from build123d import *

# Parameters (mm, degrees)
BOSS_EXTRUDE1_DEPTH = 10


with BuildPart() as part:
    # Sketch1 → Boss-Extrude1 (new body)
    with BuildSketch(Plane.XY):
        with BuildLine():
            Line((-9.709376273, 1.641432906), (-9.709376273, -21.269563621))
            Line((-9.709376273, -21.269563621), (-4.709376273, -21.269563621))
            Line((-4.709376273, -21.269563621), (-4.709376273, -13.269563621))
            Line((-4.709376273, -13.269563621), (14.600623727, -13.269563621))
            Line((14.600623727, -13.269563621), (14.600623727, -11.159563621))
            ThreePointArc((14.600623727, -11.159563621), (2.126806638, -7.715324743), (-6.812431614, 1.641432906))
            Line((-6.812431614, 1.641432906), (-9.709376273, 1.641432906))
        make_face()
        with BuildLine():
            Line((14.600623727, -11.159563621), (14.600623727, -13.269563621))
            Line((14.600623727, -13.269563621), (33.910623727, -13.269563621))
            Line((33.910623727, -13.269563621), (33.910623727, -21.269563621))
            Line((33.910623727, -21.269563621), (38.910623727, -21.269563621))
            Line((38.910623727, -21.269563621), (38.910623727, 1.641432906))
            Line((38.910623727, 1.641432906), (36.013679069, 1.641432906))
            ThreePointArc((36.013679069, 1.641432906), (27.074440817, -7.715324743), (14.600623727, -11.159563621))
        make_face()
    extrude(amount=BOSS_EXTRUDE1_DEPTH)

    # Sketch4 → CSK for M2 Countersunk Flat Head Screw1 (revolve, cut)
    with BuildSketch(Plane(origin=(-4.709376273, -17.301406974, 5), x_dir=(0, 0, -1), z_dir=(0, 1, 0))):
        Polygon((0, 0), (0, 17.221032743), (1.2, 16.5), (1.2, 1), (2.2, 0), align=None)
    csk_for_m2_countersunk_flat_head_screw1 = revolve(axis=Axis((1.640623727, -17.301406974, 5), (-1, 0, 0)), mode=Mode.SUBTRACT)

    # Mirror2: CSK for M2 Countersunk Flat Head Screw1 across plane
    add(csk_for_m2_countersunk_flat_head_screw1.mirror(Plane(origin=(14.600623727, 0, 0), x_dir=(0, 0, 1), z_dir=(1, 0, 0))), mode=Mode.SUBTRACT)


solid = part.part
The model under review builds one solid part; all positions refer to its coordinate system, in mm. A direction names the side the tool comes from. Round coordinates to 2 decimals unless told otherwise and drop trailing zeros. Order: outer loops, then holes, each group sorted by start corner. A loop starts at its lowest first (then second) coordinate and runs counter-clockwise, first axis right, second up. Notation, with made-up numbers: (12, 17.25) - (43, 17.25) arc R17 ccw to (43, 23.25) - close; hole circle Ø8 at (55, 11.25). An arc over 180 degrees is marked (long way). Use one line per item in the form item = value.
Q1. Clearance check with flat-ended pins moving along their axes: P1, Ø1.4, axis at y = -17.3, z = 5, coming from the -X side; P2, Ø1.5, axis at x = 6, z = 8, coming from the -Y side. State where each tip first meets the part, or that it passes through.
Response values:
P1 = through
P2 = -13.27
Q2. Mouldability with a two-part tool opening along X and no side actions: class faces 1 (the flat face through (-9.709, -10, 5)), 2 (the flat face through (38.911, -10, 5)), 3 (the flat face through (14, -12, 0)), 4 (the flat face through (33.911, -15, 4)) as pulls with the +X half, pulls with the -X half, needs draft (parallel to the pull), parting line crosses it, or undercut.
Response values:
face_1 = pulls with the -X half
face_2 = pulls with the +X half
face_3 = needs draft
face_4 = undercut
Q3. Add section C-C on z = 7.75. Give the boundary of the cut face in (x, y), then the cut area to 3 significant figures.
Response values:
outline = (-9.71, -21.27) - (-4.71, -21.27) - (-4.71, -13.27) - (33.91, -13.27) - (33.91, -21.27) - (38.91, -21.27) - (38.91, 1.64) - (36.01, 1.64) arc R24.31 cw to (-6.81, 1.64) - (-9.71, 1.64) - close
area = 415 mm^2
Q4. Tool access review of faces 5 (the flat face through (-4.709, -18.2, 2.7)), 6 (the flat face through (36, -21.27, 5)): name each direction out of +Z, -Z, +X, -X, +Y, -Y from which nothing blocks a thin tool from reaching the whole face with its end or side.
Response values:
face_5 = +Z, -Z, -Y
face_6 = +Z, -Z, +X, -X, -Y
Q5. Add section A-A on z = 5. Give the boundary of the cut face in (x, y).
Response values:
outline = (-9.71, -21.27) - (-4.71, -21.27) - (-4.71, -19.5) - (-5.71, -18.5) - (-9.71, -18.5) - close; (-9.71, -16.1) - (-5.71, -16.1) - (-4.71, -15.1) - (-4.71, -13.27) - (33.91, -13.27) - (33.91, -15.1) - (34.91, -16.1) - (38.91, -16.1) - (38.91, 1.64) - (36.01, 1.64) arc R24.31 cw to (-6.81, 1.64) - (-9.71, 1.64) - close; (33.91, -21.27) - (38.91, -21.27) - (38.91, -18.5) - (34.91, -18.5) - (33.91, -19.5) - close
Q6. To check wall thickness, follow line 1 (Y direction, x = 38, z = 5); line 2 (X direction, y = -18.75, z = 7.75); line 3 (X direction, y = -0.25, z = 7.5). State the ranges of each line that lie inside material, in increasing order.
Response values:
line_1 = -21.27 to -18.5, -16.1 to 1.64
line_2 = -9.71 to -4.71, 33.91 to 38.91
line_3 = -9.71 to -5.68, 34.88 to 38.91
Q7. Add section B-B on y = -4. Give the boundary of the cut face in (x, z), then the cut area to 3 significant figures.
Response values:
outline = (-9.71, 0) - (-2.63, 0) - (-2.63, 10) - (-9.71, 10) - close; (31.83, 0) - (38.91, 0) - (38.91, 10) - (31.83, 10) - close
area = 142 mm^2
Q8. Add section D-D on x = 27. Give the boundary of the cut face in (y, z).
Response values:
outline = (-13.27, 0) - (-7.76, 0) - (-7.76, 10) - (-13.27, 10) - close
